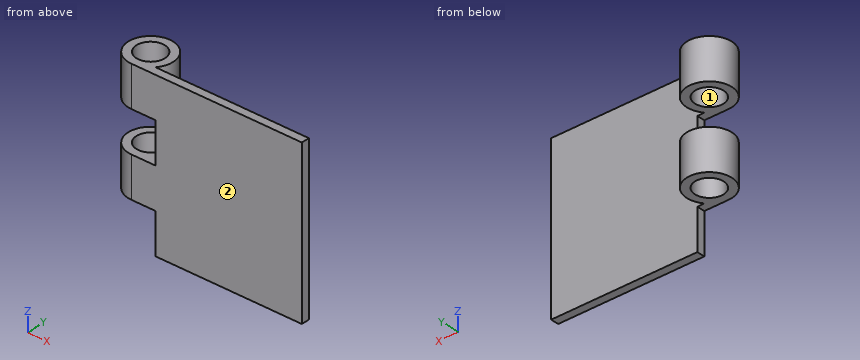
from build123d import *

# Parameters (mm, degrees)
BOSS_EXTRUDE1_DEPTH = 1
SKETCH2_R           = 2.75
SKETCH2_R_2         = 1.75
BOSS_EXTRUDE2_DEPTH = 5
BOSS_EXTRUDE3_START = -5
SKETCH3_R           = 2.75
SKETCH3_R_2         = 1.75
BOSS_EXTRUDE3_DEPTH = 5


with BuildPart() as part:
    # Sketch1 → Boss-Extrude1 (new body)
    with BuildSketch(Plane(origin=(0, 0, 0), x_dir=(1, 0, 0), z_dir=(0, 1, 0))):
        Polygon((18, 10), (18, 5), (15, 5), (15, 0), (18, 0), (18, -5), (15, -5), (15, -10), (36, -10), (36, 10), align=None)
    extrude(amount=-BOSS_EXTRUDE1_DEPTH)

    # Sketch2 → Boss-Extrude2 (add)
    with BuildSketch(Plane.XY.offset(10)):
        with Locations((15, 1.75)):
            Circle(SKETCH2_R)
        with Locations((15, 1.75)):
            Circle(SKETCH2_R_2, mode=Mode.SUBTRACT)
    extrude(amount=-BOSS_EXTRUDE2_DEPTH)

    # Sketch3 → Boss-Extrude3 (add)
    with BuildSketch(Plane(origin=(0, 0, -5), x_dir=(-1, 0, 0), z_dir=(0, 0, -1)).offset(BOSS_EXTRUDE3_START)):
        with Locations((-15, 1.75)):
            Circle(SKETCH3_R)
        with Locations(Location((-15, 1.75, 0), (0, 0, 180))):
            Circle(SKETCH3_R_2, mode=Mode.SUBTRACT)
    extrude(amount=BOSS_EXTRUDE3_DEPTH)


solid = part.part
Geometry: final body of the model. Coordinates: model frame, mm. Face numbers are marked on the shaded views. Coordinates: 2 decimals unless noted, no trailing zeros. Order: outer loops, then holes, each group sorted by start corner. A loop starts at its lowest first (then second) coordinate and runs counter-clockwise, first axis right, second up. Notation, with made-up numbers: M 54,37 L 111,37 A20 ccw 111,61 Z; hole C 47.5,-7.5 d2. An arc over 180 degrees is marked long. One line per question, with ' | ' between items. Start each with the question number.
Item 1: Pin query (flat end, axial travel): pin 1 Ø6 at (x, z) = (21, 1) entering from +Y; pin 2 Ø0.8 at (y, z) = (-0.5, -8) entering from -X; pin 3 Ø1 at (y, z) = (1, 5) entering from -X; pin 4 Ø3 at (x, y) = (30, 0.5) entering from -Z. Return the tip coordinate at first contact, or that it passes through.
Item 2: Cut plane B-B, the plane z = -3. Return the cut outline in (x, y).
Item 3: Cut plane D-D, the plane x = 33. Return the cut outline in (y, z).
Item 4: Ray query, probe 1 along Y at (x, z) = (15, -1.75); probe 2 along Y at (x, z) = (28.25, -6.25); probe 3 along X at (y, z) = (3.3, 9). Return the intervals inside material, ascending. Write a range as [from, to].
Item 5: Draft query along Y for the marked faces 1 and 2. Return one class per face: released by +Y, released by -Y, zero draft, split by the parting line, or undercut.
Item 6: Cut plane C-C, the plane y = 1.75. Return the cut outline in (x, z), then the cut area to 3 significant figures.
Item 7: Cut plane A-A, the plane y = 2.9. Return the cut outline in (x, z).
A:
1) pin 1: stops at y = 0 | pin 2: stops at x = 18 | pin 3: stops at x = 12.26 | pin 4: stops at z = -10
2) outline: M 15,-1 L 36,-1 L 36,0 L 17.12,0 A2.75 ccw long Z; hole C 15,1.75 d3.5
3) outline: M -1,-10 L 0,-10 L 0,10 L -1,10 Z
4) probe 1: y = [-1, 0], [3.5, 4.5] | probe 2: y = [-1, 0] | probe 3: x = [12.73, 14.19], [15.81, 17.27]
5) face 1: undercut | face 2: released by -Y
6) outline: M 12.25,-5 L 13.25,-5 L 13.25,0 L 12.25,0 Z; M 12.25,5 L 13.25,5 L 13.25,10 L 12.25,10 Z; M 16.75,-5 L 17.75,-5 L 17.75,0 L 16.75,0 Z; M 16.75,5 L 17.75,5 L 17.75,10 L 16.75,10 Z | area: 20.0 mm2
7) outline: M 12.5,-5 L 13.68,-5 L 13.68,0 L 12.5,0 Z; M 12.5,5 L 13.68,5 L 13.68,10 L 12.5,10 Z; M 16.32,-5 L 17.5,-5 L 17.5,0 L 16.32,0 Z; M 16.32,5 L 17.5,5 L 17.5,10 L 16.32,10 Z
